Here's how the part is built. I have some questions about the finished solid (model axes, mm). Give positions to 0.01 mm unless a question says otherwise; leave off trailing zeros. Use one line per item in the form item = value.
from build123d import *

# Parameters (mm, degrees)
SKETCH_1_R      = 2.5
EXTRUDE_1_DEPTH = 335


with BuildPart() as part:
    # 草图1 → 凸台-拉伸1 (new body)
    with BuildSketch(Plane.XY):
        with BuildLine():
            Line((4.215995631, 3.244230202), (6.436655803, 5.464890373))
            Line((6.436655803, 5.464890373), (7.776655803, 5.464890373))
            ThreePointArc((7.776655803, 5.464890373), (7.988787838, 5.377022408), (8.076655803, 5.164890373))
            Line((8.076655803, 5.164890373), (8.076655803, 3.364890373))
            ThreePointArc((8.076655803, 3.364890373), (8.164523769, 3.152758339), (8.376655803, 3.064890373))
            Line((8.376655803, 3.064890373), (9.376655803, 3.064890373))
            Line((9.376655803, 3.064890373), (9.376655803, 3.364890373))
            ThreePointArc((9.376655803, 3.364890373), (9.435234447, 3.50631173), (9.576655803, 3.564890373))
            Line((9.576655803, 3.564890373), (9.876655803, 3.564890373))
            Line((9.876655803, 3.564890373), (9.876655803, 8.464890373))
            ThreePointArc((9.876655803, 8.464890373), (9.437315975, 9.525550545), (8.376655803, 9.964890373))
            Line((8.376655803, 9.964890373), (3.476655803, 9.964890373))
            Line((3.476655803, 9.964890373), (3.476655803, 9.664890373))
            ThreePointArc((3.476655803, 9.664890373), (3.418077159, 9.523469017), (3.276655803, 9.464890373))
            Line((3.276655803, 9.464890373), (2.976655803, 9.464890373))
            Line((2.976655803, 9.464890373), (2.976655803, 8.464890373))
            ThreePointArc((2.976655803, 8.464890373), (3.064523769, 8.252758339), (3.276655803, 8.164890373))
            Line((3.276655803, 8.164890373), (5.076655803, 8.164890373))
            ThreePointArc((5.076655803, 8.164890373), (5.288787838, 8.077022408), (5.376655803, 7.864890373))
            Line((5.376655803, 7.864890373), (5.376655803, 6.524890373))
            Line((5.376655803, 6.524890373), (3.155995631, 4.304230202))
            ThreePointArc((3.155995631, 4.304230202), (2.669360608, 3.979071075), (2.09533546, 3.864890373))
            Line((2.09533546, 3.864890373), (-2.342023853, 3.864890373))
            ThreePointArc((-2.342023853, 3.864890373), (-2.916049002, 3.979071075), (-3.402684025, 4.304230202))
            Line((-3.402684025, 4.304230202), (-5.623344197, 6.524890373))
            Line((-5.623344197, 6.524890373), (-5.623344197, 7.864890373))
            ThreePointArc((-5.623344197, 7.864890373), (-5.535476231, 8.077022408), (-5.323344197, 8.164890373))
            Line((-5.323344197, 8.164890373), (-3.523344197, 8.164890373))
            ThreePointArc((-3.523344197, 8.164890373), (-3.311212162, 8.252758339), (-3.223344197, 8.464890373))
            Line((-3.223344197, 8.464890373), (-3.223344197, 9.464890373))
            Line((-3.223344197, 9.464890373), (-3.523344197, 9.464890373))
            ThreePointArc((-3.523344197, 9.464890373), (-3.664765553, 9.523469017), (-3.723344197, 9.664890373))
            Line((-3.723344197, 9.664890373), (-3.723344197, 9.964890373))
            Line((-3.723344197, 9.964890373), (-8.623344197, 9.964890373))
            ThreePointArc((-8.623344197, 9.964890373), (-9.684004369, 9.525550545), (-10.123344197, 8.464890373))
            Line((-10.123344197, 8.464890373), (-10.123344197, 3.564890373))
            Line((-10.123344197, 3.564890373), (-9.823344197, 3.564890373))
            ThreePointArc((-9.823344197, 3.564890373), (-9.681922841, 3.50631173), (-9.623344197, 3.364890373))
            Line((-9.623344197, 3.364890373), (-9.623344197, 3.064890373))
            Line((-9.623344197, 3.064890373), (-8.623344197, 3.064890373))
            ThreePointArc((-8.623344197, 3.064890373), (-8.411212162, 3.152758339), (-8.323344197, 3.364890373))
            Line((-8.323344197, 3.364890373), (-8.323344197, 5.164890373))
            ThreePointArc((-8.323344197, 5.164890373), (-8.235476231, 5.377022408), (-8.023344197, 5.464890373))
            Line((-8.023344197, 5.464890373), (-6.683344197, 5.464890373))
            Line((-6.683344197, 5.464890373), (-4.462684025, 3.244230202))
            ThreePointArc((-4.462684025, 3.244230202), (-4.137524898, 2.757595178), (-4.023344197, 2.18357003))
            Line((-4.023344197, 2.18357003), (-4.023344197, -2.253789283))
            ThreePointArc((-4.023344197, -2.253789283), (-4.137524898, -2.827814432), (-4.462684025, -3.314449455))
            Line((-4.462684025, -3.314449455), (-6.683344197, -5.535109627))
            Line((-6.683344197, -5.535109627), (-8.023344197, -5.535109627))
            ThreePointArc((-8.023344197, -5.535109627), (-8.235476231, -5.447241661), (-8.323344197, -5.235109627))
            Line((-8.323344197, -5.235109627), (-8.323344197, -3.435109627))
            ThreePointArc((-8.323344197, -3.435109627), (-8.411212162, -3.222977592), (-8.623344197, -3.135109627))
            Line((-8.623344197, -3.135109627), (-9.623344197, -3.135109627))
            Line((-9.623344197, -3.135109627), (-9.623344197, -3.435109627))
            ThreePointArc((-9.623344197, -3.435109627), (-9.681922841, -3.576530983), (-9.823344197, -3.635109627))
            Line((-9.823344197, -3.635109627), (-10.123344197, -3.635109627))
            Line((-10.123344197, -3.635109627), (-10.123344197, -8.535109627))
            ThreePointArc((-10.123344197, -8.535109627), (-9.684004369, -9.595769798), (-8.623344197, -10.035109627))
            Line((-8.623344197, -10.035109627), (-3.723344197, -10.035109627))
            Line((-3.723344197, -10.035109627), (-3.723344197, -9.735109627))
            ThreePointArc((-3.723344197, -9.735109627), (-3.664765553, -9.59368827), (-3.523344197, -9.535109627))
            Line((-3.523344197, -9.535109627), (-3.223344197, -9.535109627))
            Line((-3.223344197, -9.535109627), (-3.223344197, -8.535109627))
            ThreePointArc((-3.223344197, -8.535109627), (-3.311212162, -8.322977592), (-3.523344197, -8.235109627))
            Line((-3.523344197, -8.235109627), (-5.323344197, -8.235109627))
            ThreePointArc((-5.323344197, -8.235109627), (-5.535476231, -8.147241661), (-5.623344197, -7.935109627))
            Line((-5.623344197, -7.935109627), (-5.623344197, -6.595109627))
            Line((-5.623344197, -6.595109627), (-3.402684025, -4.374449455))
            ThreePointArc((-3.402684025, -4.374449455), (-2.916049002, -4.049290328), (-2.342023853, -3.935109627))
            Line((-2.342023853, -3.935109627), (2.09533546, -3.935109627))
            ThreePointArc((2.09533546, -3.935109627), (2.669360608, -4.049290328), (3.155995631, -4.374449455))
            Line((3.155995631, -4.374449455), (5.376655803, -6.595109627))
            Line((5.376655803, -6.595109627), (5.376655803, -7.935109627))
            ThreePointArc((5.376655803, -7.935109627), (5.288787838, -8.147241661), (5.076655803, -8.235109627))
            Line((5.076655803, -8.235109627), (3.276655803, -8.235109627))
            ThreePointArc((3.276655803, -8.235109627), (3.064523769, -8.322977592), (2.976655803, -8.535109627))
            Line((2.976655803, -8.535109627), (2.976655803, -9.535109627))
            Line((2.976655803, -9.535109627), (3.276655803, -9.535109627))
            ThreePointArc((3.276655803, -9.535109627), (3.418077159, -9.59368827), (3.476655803, -9.735109627))
            Line((3.476655803, -9.735109627), (3.476655803, -10.035109627))
            Line((3.476655803, -10.035109627), (8.376655803, -10.035109627))
            ThreePointArc((8.376655803, -10.035109627), (9.437315975, -9.595769798), (9.876655803, -8.535109627))
            Line((9.876655803, -8.535109627), (9.876655803, -3.635109627))
            Line((9.876655803, -3.635109627), (9.576655803, -3.635109627))
            ThreePointArc((9.576655803, -3.635109627), (9.435234447, -3.576530983), (9.376655803, -3.435109627))
            Line((9.376655803, -3.435109627), (9.376655803, -3.135109627))
            Line((9.376655803, -3.135109627), (8.376655803, -3.135109627))
            ThreePointArc((8.376655803, -3.135109627), (8.164523769, -3.222977592), (8.076655803, -3.435109627))
            Line((8.076655803, -3.435109627), (8.076655803, -5.235109627))
            ThreePointArc((8.076655803, -5.235109627), (7.988787838, -5.447241661), (7.776655803, -5.535109627))
            Line((7.776655803, -5.535109627), (6.436655803, -5.535109627))
            Line((6.436655803, -5.535109627), (4.215995631, -3.314449455))
            ThreePointArc((4.215995631, -3.314449455), (3.890836504, -2.827814432), (3.776655803, -2.253789283))
            Line((3.776655803, -2.253789283), (3.776655803, 2.18357003))
            ThreePointArc((3.776655803, 2.18357003), (3.890836504, 2.757595178), (4.215995631, 3.244230202))
        make_face()
        with Locations((-0.123344197, -0.035109627)):
            Circle(SKETCH_1_R, mode=Mode.SUBTRACT)
    extrude(amount=EXTRUDE_1_DEPTH)


solid = part.part
(1) Thinking about a two-plate mould opening in Z: for faces 1 (the flat face through (2, 2, 335)), 2 (the flat face through (2, 2, 0)), which applies, pulls with the +Z half, pulls with the -Z half, needs draft (parallel to the pull), parting line crosses it, or undercut?
Geometry says:
face_1 = pulls with the +Z half
face_2 = pulls with the -Z half
(2) For P1, Ø5, axis at y = 0.5, z = 179.5, coming from the +X side; P2, Ø2, axis at x = -3.5, z = 176.5, coming from the -Y side, each with a flat end and sliding along its axis, tell me the tip position at first contact or that it passes through.
Geometry says:
P1 = 4.02
P2 = -10.04
(3) If I drill on probe 1 along X at (y, z) = (4.25, 49); probe 2 along Y at (x, z) = (4.25, 241.5); probe 3 along X at (y, z) = (3.5, 160.5), over which ranges is the centre line in solid material (lowest first)?
Geometry says:
probe_1 = -10.12 to -8.32, -5.47 to -3.35, 3.1 to 5.22, 8.08 to 9.88
probe_2 = -10.04 to -8.24, -5.47 to -3.35, 3.28 to 5.4, 8.16 to 9.96
probe_3 = -9.68 to -8.32, -4.72 to 4.47, 8.08 to 9.43
